Geometry: see drawing. Coordinates: mm, zero at the bounding-box minimum. Give positions to 0.01 mm unless a question says otherwise; leave off trailing zeros. Write each loop counter-clockwise with the first axis right and the second up, starting at its lowest first coordinate (ties: lowest second). Pieces come first, ordered by that corner, then holes. Notation, with made-up numbers: M 16,-21 L 57,-21 A22 cw 57,3 Z; hole C 22,89 d7. An arc over 180 degrees is marked long. Use a Markdown table: item, result. Add a question column.
(1) Cut plane A-A (y = 33.5). Output: boundary loops of the cut face in (x, z), plus the area to 3 significant figures.
(2) Material intervals for L1, parallel to Y at x = 47, z = 1.75; L2, parallel to X at y = 7.5, z = 1.75; L3, parallel to X at y = 7, z = 1, sorted ascending.
(3) Pin query (flat end, axial travel): pin 1 Ø1 at (y, z) = (22.5, 3.5) entering from +X. Return the tip coordinate at first contact, or that it passes through.
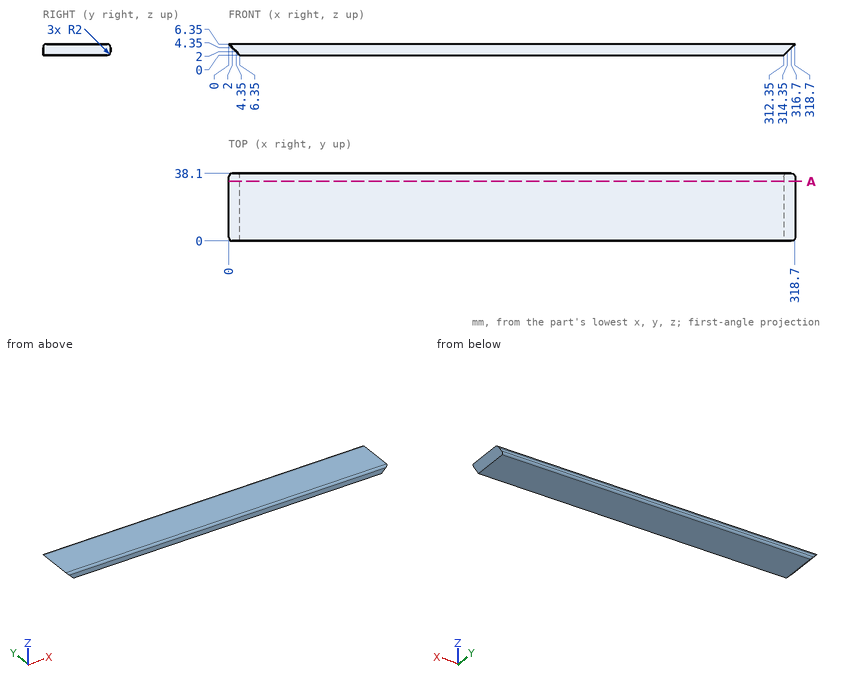
Answer list:
| question | item | result |
|---|---|---|
| 1 | outline | M 0,6.35 L 6.35,0 L 312.35,0 L 318.7,6.35 Z |
| 1 | area | 1,980 mm² |
| 2 | L1 | 0 to 38.08 |
| 2 | L2 | 4.6 to 314.1 |
| 2 | L3 | 5.35 to 313.35 |
| 3 | pin 1 | x = 316.35 |
